Source: CAD feature listing. Evaluate the final solid. Frame: model axes, mm. A direction names the side the tool comes from. Coordinates: 2 decimals unless noted, no trailing zeros. Order: outer loops, then holes, each group sorted by start corner. A loop starts at its lowest first (then second) coordinate and runs counter-clockwise, first axis right, second up.
```python
from build123d import *

# Parameters (mm, degrees)
F0_W          = 100
F0_H          = 40
F1_DEPTH      = 10
F3_DEPTH      = 10
F4_W          = 40
F4_H          = 3
F5_DEPTH      = 40.001
F6_R          = 2.25
F7_DEPTH      = 40.001
F8_R          = 4.5
F9_DEPTH      = 5.7
F10_T1_DEPTH  = 40
F10_T3_DEPTH  = 40
F10_T5_DEPTH  = 50
F10_T7_DEPTH  = 50
F10_T9_DEPTH  = 50
F10_T11_DEPTH = 50
F11_F1_R      = 3
F11_F2_R      = 3
F11_F3_R      = 3


# Not quite as in the source:
# - a fillet or chamfer that OpenCascade refuses, or shapes differently, is made with other operations: its cross-section is extruded or revolved along the edge and cut away or added


with BuildPart() as f1:
    # F0 (on Front) → F1 (new body)
    with BuildSketch(Plane.XZ):
        with Locations((50, 20)):
            Rectangle(F0_W, F0_H)
    extrude(amount=F1_DEPTH)

    # F2 (on Top) → F3 (join)
    with BuildSketch(Plane.XY):
        with BuildLine():
            Line((70, 0), (30, 0))
            Line((30, 0), (30, -35))
            ThreePointArc((30, -35), (50, -55), (70, -35))
            Line((70, -35), (70, 0))
        make_face()
    extrude(amount=F3_DEPTH)

    # F4 (on face) → F5 (cut, through all)
    with BuildSketch(Plane(origin=(0, 0, 0), x_dir=(1, 0, 0), z_dir=(0, 0, -1))):
        with Locations((50, 1.5)):
            Rectangle(F4_W, F4_H)
    extrude(amount=-F5_DEPTH, mode=Mode.SUBTRACT)

    # F6 (on face) → F7 (cut, through all)
    with BuildSketch(Plane(origin=(0, 0, 0), x_dir=(1, 0, 0), z_dir=(0, 0, -1))):
        with Locations((50, 35)):
            Circle(F6_R)
    extrude(amount=-F7_DEPTH, mode=Mode.SUBTRACT)

    # F8 (on face) → F9 (cut)
    with BuildSketch(Plane(origin=(0, 0, 0), x_dir=(1, 0, 0), z_dir=(0, 0, -1))):
        with Locations((50, 35)):
            Circle(F8_R)
    extrude(amount=-F9_DEPTH, mode=Mode.SUBTRACT)

    # F10: fillet of radius 8 on 6 edges, made by hand

    # F10_s2 → F10_t1 (join)
    with BuildSketch(Plane.XY):
        with BuildLine():
            ThreePointArc((70, 0), (67.2191036167, -2.2111025509), (63.7550020016, -3))
            Line((63.7550020016, -3), (70, -3))
            Line((70, -3), (70, 0))
        make_face()
    extrude(amount=F10_T1_DEPTH)

    # F10_s4 → F10_t3 (join)
    with BuildSketch(Plane.XY):
        with BuildLine():
            ThreePointArc((36.2449979984, -3), (32.7808963833, -2.2111025509), (30, 0))
            Line((30, 0), (30, -3))
            Line((30, -3), (36.2449979984, -3))
        make_face()
    extrude(amount=F10_T3_DEPTH)

    # F10_s6 → F10_t5 (cut)
    with BuildSketch(Plane.XZ.offset(-20)):
        with BuildLine():
            ThreePointArc((0, 32), (2.3431457505, 37.6568542495), (8, 40))
            Line((8, 40), (0, 40))
            Line((0, 40), (0, 32))
        make_face()
    extrude(amount=F10_T5_DEPTH, mode=Mode.SUBTRACT)

    # F10_s8 → F10_t7 (cut)
    with BuildSketch(Plane.XZ.offset(-20)):
        with BuildLine():
            ThreePointArc((0, 8), (2.3431457505, 2.3431457505), (8, 0))
            Line((8, 0), (0, 0))
            Line((0, 0), (0, 8))
        make_face()
    extrude(amount=F10_T7_DEPTH, mode=Mode.SUBTRACT)

    # F10_s10 → F10_t9 (cut)
    with BuildSketch(Plane.XZ.offset(-20)):
        with BuildLine():
            ThreePointArc((92, 40), (97.6568542495, 37.6568542495), (100, 32))
            Line((100, 32), (100, 40))
            Line((100, 40), (92, 40))
        make_face()
    extrude(amount=F10_T9_DEPTH, mode=Mode.SUBTRACT)

    # F10_s12 → F10_t11 (cut)
    with BuildSketch(Plane.XZ.offset(-20)):
        with BuildLine():
            ThreePointArc((92, 0), (97.6568542495, 2.3431457505), (100, 8))
            Line((100, 8), (100, 0))
            Line((100, 0), (92, 0))
        make_face()
    extrude(amount=F10_T11_DEPTH, mode=Mode.SUBTRACT)

    # F11: fillet of radius 3 on 17 edges, made by hand

    # F11_f1
    f11_f1_edges = [f1.edges().sort_by_distance(p)[0] for p in [
        (50, -55, 10),
        (70, -22.5, 10),
        (30, -22.5, 10),
    ]]
    fillet(f11_f1_edges, radius=F11_F1_R)

    # F11_f2
    f11_f2_edges = [f1.edges().sort_by_distance(p)[0] for p in [
        (70, -10, 3.5),
        (50, -10, 10),
        (69.1213203436, -10, 9.1213203436),
        (30.8786796564, -10, 9.1213203436),
    ]]
    fillet(f11_f2_edges, radius=F11_F2_R)

    # F11_f3
    f11_f3_edges = [f1.edges().sort_by_distance(p)[0] for p in [
        (50, -55, 0),
        (0, -10, 20),
        (2.3431457505, -10, 2.3431457505),
        (17.5, -10, 0),
        (2.3431457505, -10, 37.6568542495),
        (50, -10, 40),
        (97.6568542495, -10, 37.6568542495),
        (100, -10, 20),
        (97.6568542495, -10, 2.3431457505),
        (82.5, -10, 0),
        (70, -24, 0),
        (30, -24, 0),
        (29.1213203436, -10.8786796564, 0),
        (70.8786796564, -10.8786796564, 0),
    ]]
    fillet(f11_f3_edges, radius=F11_F3_R)


solid = f1.part
```
1. Section query B-B on z = 26. Return loops of the section in (x, y) (3 decimals), plus the area to 3 significant figures.
Findings:
outline: (0, -7) arc R3 ccw to (3, -10) - (97, -10) arc R3 ccw to (100, -7) - (100, 0) - (70, 0) arc R8 cw to (63.755, -3) - (36.245, -3) arc R8 cw to (30, 0) - (0, 0) - close
area: 888 mm2
2. Draft query along Y for faces 6 (the face through (49, -10, 24)), 7 (the face through (52.08, -31.01, 2.81)), 8 (the face through (0, -3, 20)). Return one class per face: released by +Y, released by -Y, zero draft, split by the parting line, or undercut.
Findings:
face 6: released by -Y
face 7: undercut
face 8: zero draft
3. Access query for faces 1 (the face through (30, -24, 5)), 2 (the face through (67.26, -2.19, 19.72)), 3 (the face through (69.1, -23.85, 0.86)), 4 (the face through (17.63, -9.1, 0.86)), 5 (the face through (30.86, -24.15, 9.1)). Directions: +Z, -Z, +X, -X, +Y, -Y. A direction counts if a zero-diameter tool reaches every point of the face in a straight line with its end or side. Return the directions, or none.
Findings:
face 1: +Z, -Z, -X, -Y
face 2: +Z, -Z, +Y
face 3: -Z, +X, -Y
face 4: -Z, -X, -Y
face 5: +Z, -X, -Y
4. Pin query (flat end, axial travel): P1, Ø10, axis at x = 64.5, z = 9.5, coming from the -Y side; P2, Ø7, axis at x = 50, y = -35, coming from the -Z side; P3, Ø2, axis at y = -24.5, z = 5.5, coming from the +X side. Return the tip coordinate at first contact, or that it passes through.
Findings:
P1: stops at y = -52.32
P2: stops at z = 5.7
P3: stops at x = 70
5. Section query A-A on x = 50. Return loops of the section in (y, z).
Findings:
outline: (-55, 3) arc R3 ccw to (-52, 0) - (-39.5, 0) - (-39.5, 5.7) - (-37.25, 5.7) - (-37.25, 10) - (-52, 10) arc R3 ccw to (-55, 7) - close; (-32.75, 5.7) - (-30.5, 5.7) - (-30.5, 0) - (-3, 0) - (-3, 40) - (-7, 40) arc R3 ccw to (-10, 37) - (-10, 13) arc R3 cw to (-13, 10) - (-32.75, 10) - close
6. Ray query, line 1 (X direction, y = -35, z = 2.85); line 2 (Y direction, x = 50, z = 4); line 3 (Z direction, x = 44.5, y = -39). Return the intervals inside material, ascending.
Findings:
line 1: x = 30 to 45.5, 54.5 to 70
line 2: y = -55 to -39.5, -30.5 to -3
line 3: z = 0 to 10
7. Section query C-C on x = 79. Return loops of the section in (y, z), plus the area to 3 significant figures.
Findings:
outline: (-10, 3) arc R3 ccw to (-7, 0) - (0, 0) - (0, 40) - (-7, 40) arc R3 ccw to (-10, 37) - close
area: 396 mm2
